CAD build for the part. Positions are in the model's coordinates, mm. A direction names the side the tool comes from. Give positions to 0.01 mm unless a question says otherwise; leave off trailing zeros. Loops run counter-clockwise (first coordinate to the right, second up) from the corner with the lowest first, then second, coordinate; pieces in that order, holes last. Notation, with made-up numbers: (73, -8.5) -> (119, -8.5) arc R24 cw to (119, 2.5) -> close; hole circle Ø6 at (-29.75, -24.75). An arc over 180 degrees is marked (long way). Use one line per item in the form item = value.
```python
from build123d import *

# Parameters (mm, degrees)
BOSS_EXTRUDE1_DEPTH = 50.8
SKETCH1_4_W         = 13.934163053
SKETCH1_4_H         = 71.12
BOSS_EXTRUDE2_DEPTH = 50.8
CUT_EXTRUDE1_START  = -32.984163053
CUT_EXTRUDE1_DEPTH  = 65.968326106
SKETCH3_R           = 3.937
SKETCH3_W           = 2.54
SKETCH3_H           = 10.16
CUT_EXTRUDE2_DEPTH  = 8.255
SKETCH3_2_W         = 2.54
SKETCH3_2_H         = 10.16
CUT_EXTRUDE3_DEPTH  = 28.255
CUT_EXTRUDE4_START  = 32.984163
CUT_EXTRUDE4_DEPTH  = 10.775
CUT_EXTRUDE5_START  = -22.209163
CUT_EXTRUDE5_DEPTH  = 10.775
FILLET1_R           = 10


# Read off the part's stored shape, not the designer's step: Cut-Extrude1
with BuildPart() as part:
    # Sketch1 → Boss-Extrude1 (new body)
    with BuildSketch(Plane(origin=(0, 0, 0), x_dir=(1, 0, 0), z_dir=(0, 1, 0))):
        with BuildLine():
            ThreePointArc((13.97, 0), (0, -13.97), (-13.97, 0))
            Line((-13.97, 0), (-32.984163053, 0))
            Line((-32.984163053, 0), (-32.984163053, -25.4))
            Line((-32.984163053, -25.4), (-19.05, -25.4))
            Line((-19.05, -25.4), (19.05, -25.4))
            Line((19.05, -25.4), (32.984163053, -25.4))
            Line((32.984163053, -25.4), (32.984163053, 0))
            Line((32.984163053, 0), (13.97, 0))
        make_face()
    extrude(amount=BOSS_EXTRUDE1_DEPTH)

    # Sketch1<4> → Boss-Extrude2 (add)
    with BuildSketch(Plane(origin=(0, 0, 0), x_dir=(1, 0, 0), z_dir=(0, 1, 0))):
        with Locations((-26.017081527, -60.96)):
            Rectangle(SKETCH1_4_W, SKETCH1_4_H)
        with Locations((26.017081527, -60.96)):
            Rectangle(SKETCH1_4_W, SKETCH1_4_H)
    extrude(amount=BOSS_EXTRUDE2_DEPTH)

    # Cut-Extrude1 outline → Cut-Extrude1 (cut)
    with BuildSketch(Plane(origin=(0, 0, 0), x_dir=(0, 0, -1), z_dir=(1, 0, 0)).offset(CUT_EXTRUDE1_START)):
        Polygon((-96.52, 0), (-25.4, 0), (-96.52, 19.05), align=None)
        Polygon((-91.52, 31.75), (-25.4, 31.75), (-25.4, 50.8), (-96.52, 50.8), (-96.52, 36.75), (-91.52, 36.75), align=None)
    extrude(amount=CUT_EXTRUDE1_DEPTH, mode=Mode.SUBTRACT)

    # Sketch3 → Cut-Extrude2 (cut)
    with BuildSketch(Plane.XY):
        with Locations((23.479163053, 25.4)):
            Circle(SKETCH3_R)
        with Locations((-23.479163053, 25.4)):
            Circle(SKETCH3_R)
        with Locations((23.479163053, 35.48)):
            Rectangle(SKETCH3_W, SKETCH3_H)
        with Locations((-23.479163053, 35.48)):
            Rectangle(SKETCH3_W, SKETCH3_H)
        with Locations((-23.479163053, 15.32)):
            Rectangle(SKETCH3_W, SKETCH3_H)
        with Locations((23.479163053, 15.32)):
            Rectangle(SKETCH3_W, SKETCH3_H)
    extrude(amount=CUT_EXTRUDE2_DEPTH, mode=Mode.SUBTRACT)

    # Sketch3<2> → Cut-Extrude3 (cut)
    with BuildSketch(Plane.XY):
        with Locations((23.479163053, 35.48)):
            Rectangle(SKETCH3_2_W, SKETCH3_2_H)
        with Locations((-23.479163053, 35.48)):
            Rectangle(SKETCH3_2_W, SKETCH3_2_H)
        with Locations((23.479163053, 15.32)):
            Rectangle(SKETCH3_2_W, SKETCH3_2_H)
        with Locations((-23.479163053, 15.32)):
            Rectangle(SKETCH3_2_W, SKETCH3_2_H)
    extrude(amount=CUT_EXTRUDE3_DEPTH, mode=Mode.SUBTRACT)

    # Sketch2<4> → Cut-Extrude4 (cut)
    with BuildSketch(Plane(origin=(0, 0, 0), x_dir=(0, 0, -1), z_dir=(1, 0, 0)).offset(CUT_EXTRUDE4_START)):
        Polygon((-22.4, 20.4), (-25.4, 20.4), (-25.4, 19.05), (-25.4, 10.24), (-22.4, 10.24), align=None)
    extrude(amount=-CUT_EXTRUDE4_DEPTH, mode=Mode.SUBTRACT)

    # Sketch2<5> → Cut-Extrude5 (cut)
    with BuildSketch(Plane(origin=(0, 0, 0), x_dir=(0, 0, -1), z_dir=(1, 0, 0)).offset(CUT_EXTRUDE5_START)):
        Polygon((-22.4, 20.4), (-25.4, 20.4), (-25.4, 19.05), (-25.4, 10.24), (-22.4, 10.24), align=None)
    extrude(amount=-CUT_EXTRUDE5_DEPTH, mode=Mode.SUBTRACT)

    # Fillet1
    # the kernel refuses this fillet: 10 mm, written as the material it adds along each edge
    with BuildSketch(Plane(origin=(22.209163053, 10.24, 28.255), x_dir=(0, 0, -1), z_dir=(0, 1, 0)), Plane(origin=(-22.209163053, 20.4, 28.255), x_dir=(0, 0, -1), z_dir=(0, -1, 0))) as fillet1_piece_1:
        with BuildLine():
            CenterArc((6.659459438, -10), FILLET1_R, 90, 41.754936598)
            Line((0, -2.54), (0, 0))
            Line((0, 0), (6.659459438, 0))
        make_face()
    extrude(amount=10.16)
    # the kernel refuses this fillet: 10 mm, written as the material it takes off along each edge
    with BuildSketch(Plane(origin=(-24.749163053, 20.4, 22.4), x_dir=(0, 0, -1), z_dir=(0, -1, 0))) as fillet1_2_piece_1:
        with BuildLine():
            CenterArc((9.843006391, -10), FILLET1_R, 90, 79.834039024)
            Line((0, -8.234999947), (0, 0))
            Line((0, 0), (9.843006391, 0))
        make_face()
    extrude(amount=10.16, mode=Mode.SUBTRACT)
    with BuildSketch(Plane(origin=(24.749163053, 20.4, 22.4), x_dir=(0, 0, -1), z_dir=(0, -1, 0))) as fillet1_2_piece_2:
        with BuildLine():
            CenterArc((9.843006391, 10), FILLET1_R, 190.165960976, 79.834039024)
            Line((0, 8.234999947), (0, 0))
            Line((0, 0), (9.843006391, 0))
        make_face()
    extrude(amount=10.16, mode=Mode.SUBTRACT)


solid = part.part
```
1. Cut at C-C, the plane y = 25.4. Write the cut outline in (x, z) (3 decimals), then the cut area to 3 significant figures.
Result sheet:
outline = (-32.984, 0) -> (-27.416, 0) -> (-27.416, 8.255) -> (-19.542, 8.255) -> (-19.542, 0) -> (-13.97, 0) arc R13.97 cw to (13.97, 0) -> (19.542, 0) -> (19.542, 8.255) -> (27.416, 8.255) -> (27.416, 0) -> (32.984, 0) -> (32.984, 96.52) -> (19.05, 96.52) -> (19.05, 25.4) -> (-19.05, 25.4) -> (-19.05, 96.52) -> (-32.984, 96.52) -> close
area = 3,220 mm^2
2. Drill centre lines: line 1 (X direction, y = 31.5, z = 79.5); line 2 (Z direction, x = 26.5, y = 26.5) (3 decimals); line 3 (X direction, y = 25, z = 2). Where is each one in solid material? Low to high.
Result sheet:
line_1 = -32.98 to -19.05, 19.05 to 32.98
line_2 = 8.255 to 96.52
line_3 = -32.98 to -27.4, -19.56 to -13.83, 13.83 to 19.56, 27.4 to 32.98
3. Cut at B-B, the plane z = 44.5. Write the cut outline in (x, y).
Result sheet:
outline = (-32.98, 5.12) -> (-19.05, 5.12) -> (-19.05, 31.75) -> (-32.98, 31.75) -> close; (19.05, 5.12) -> (32.98, 5.12) -> (32.98, 31.75) -> (19.05, 31.75) -> close
4. Cut at D-D, the plane x = 0. Write the cut outline in (y, z), then the cut area to 3 significant figures.
Result sheet:
outline = (0, 13.97) -> (50.8, 13.97) -> (50.8, 25.4) -> (0, 25.4) -> close
area = 581 mm^2
5. Mould opens along Z. For faces 1 (the flat face through (26, 31.75, 59)), 2 (the flat face through (-26, 28, 96.52)), 3 (the flat face through (-26, 36.75, 94)) say: pulls with the +Z half, pulls with the -Z half, needs draft (parallel to the pull), parting line crosses it, or undercut.
Result sheet:
face_1 = undercut
face_2 = pulls with the +Z half
face_3 = needs draft
6. Drop flat-ended pins along their axis: P1, Ø15, axis at x = 9, y = 25.5, coming from the +Z side; P2, Ø15.5, axis at x = 23.5, z = 70.5, coming from the +Y side. Give the stop position or say it passes through.
Result sheet:
P1 = 25.4
P2 = 31.75
7. Cut at A-A, the plane y = 13.5. Write the cut outline in (x, z) (3 decimals).
Result sheet:
outline = (-32.984, 0) -> (-24.749, 0) -> (-24.749, 12.557) arc R10 ccw to (-32.984, 22.4) -> close; (-32.984, 25.4) -> (-24.749, 25.4) -> (-24.749, 28.255) arc R10 cw to (-22.209, 21.596) -> (-22.209, 0) -> (-13.97, 0) arc R13.97 cw to (13.97, 0) -> (22.209, 0) -> (22.209, 21.596) arc R10 cw to (24.749, 28.255) -> (24.749, 25.4) -> (32.984, 25.4) -> (32.984, 75.8) -> (19.05, 75.8) -> (19.05, 25.4) -> (-19.05, 25.4) -> (-19.05, 75.8) -> (-32.984, 75.8) -> close; (24.749, 0) -> (32.984, 0) -> (32.984, 22.4) arc R10 ccw to (24.749, 12.557) -> close
8. Tool access for faces 4 (the flat face through (-26, 31.75, 59)), 5 (the cylindrical face through (-27.02, 15.39, 18.9)), 6 (the flat face through (26, 36.75, 94)), 7 (the flat face through (22.209, 15, 11)): list every direction of +Z, -Z, +X, -X, +Y, -Y with a clear straight run to the whole face (end or side of a thin tool).
Result sheet:
face_4 = +X, -X, +Y
face_5 = none
face_6 = +Z, +X, -X, +Y
face_7 = -Z
